Check sheet for the drawn part. Datum: minimum x, y, z corner. Units: mm. Coordinates: 2 decimals unless noted, no trailing zeros. Order: outer loops, then holes, each group sorted by start corner. A loop starts at its lowest first (then second) coordinate and runs counter-clockwise, first axis right, second up. Notation, with made-up numbers: (39, -15.75) - (45, -15.75) arc R18 ccw to (45, -6.75) - close; hole circle Ø6 at (45, 14). An arc over 180 degrees is marked (long way). Put each result on its own line as item: value.
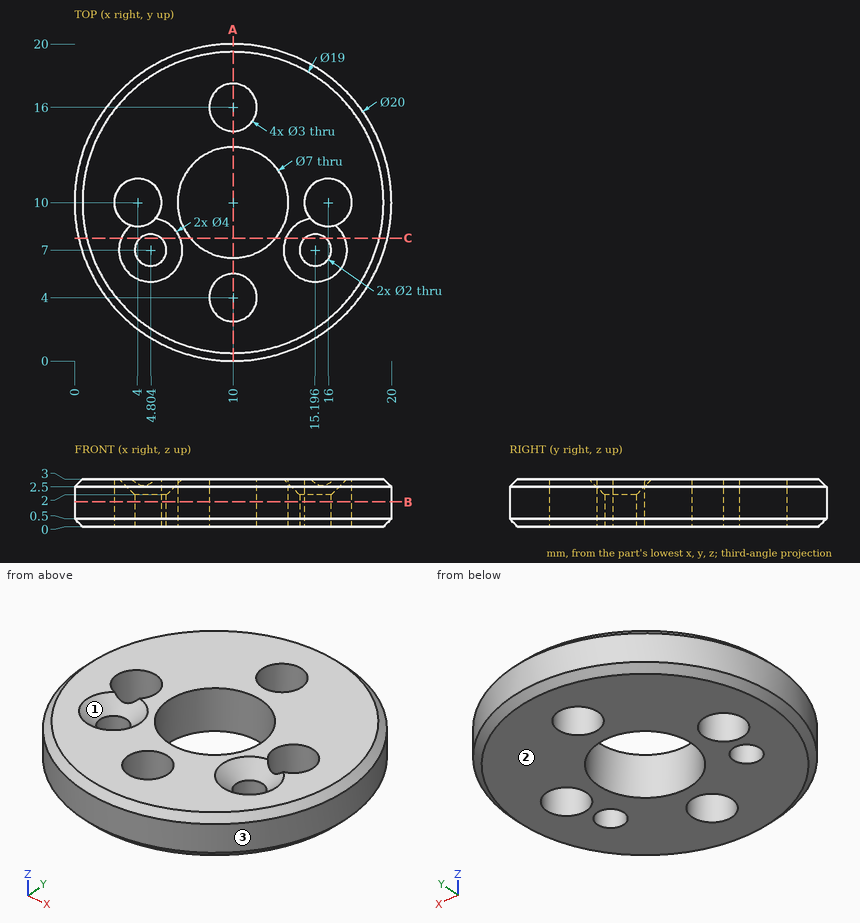
Q1. Section check B-B on z = 1.55. Record the boundary of the cut face in (x, y), then the cut area to 3 significant figures.
Answer block:
outline: circle Ø20 at (10, 10); hole circle Ø3 at (4, 10); hole circle Ø2 at (4.8, 7); hole circle Ø7 at (10, 10); hole circle Ø3 at (10, 4); hole circle Ø3 at (10, 16); hole circle Ø2 at (15.2, 7); hole circle Ø3 at (16, 10)
area: 241 mm^2
Q2. Depth check by flat-ended pin: pin 1 Ø3 at (x, y) = (4.8, 7) entering from +Z; pin 2 Ø8 at (x, y) = (17.5, 3.5) entering from +Z; pin 3 Ø1.5 at (x, z) = (9, 2) entering from -Y. Enter the tip coordinate at first touch or a pass-through.
Answer block:
pin 1: stops at z = 2.5
pin 2: stops at z = 3
pin 3: stops at y = 0
Q3. Section check A-A on x = 10. Record the boundary of the cut face in (y, z).
Answer block:
outline: (0, 0.5) - (0.5, 0) - (2.5, 0) - (2.5, 3) - (0.5, 3) - (0, 2.5) - close; (5.5, 0) - (6.5, 0) - (6.5, 3) - (5.5, 3) - close; (13.5, 0) - (14.5, 0) - (14.5, 3) - (13.5, 3) - close; (17.5, 0) - (19.5, 0) - (20, 0.5) - (20, 2.5) - (19.5, 3) - (17.5, 3) - close
Q4. Draft check along X on the marked faces 1, 2 and 3. Enter one of: pulls with the +X half, pulls with the -X half, needs draft (parallel to the pull), parting line crosses it, or undercut.
Answer block:
face 1: undercut
face 2: needs draft
face 3: parting line crosses it
Q5. Section check C-C on y = 7.75. State how many separate pieces and enclosed holes the cut face has, then the cut area to 3 significant figures.
Answer block:
separate pieces: 4
enclosed holes: 0
area: 31.4 mm^2
Q6. Thickness scan on L1, parallel to Y at x = 10, z = 0.8; L2, parallel to Y at x = 11, z = 2.1; L3, parallel to Y at x = 16, z = 1.6 (1 decimal). Record the ranges inside material, lowest first. Write a range as [from, to].
Answer block:
L1: y = [0, 2.5], [5.5, 6.5], [13.5, 14.5], [17.5, 20]
L2: y = [0.05, 2.88], [5.12, 6.65], [13.35, 14.88], [17.12, 19.95]
L3: y = [2, 6.4], [7.6, 8.5], [11.5, 18]
